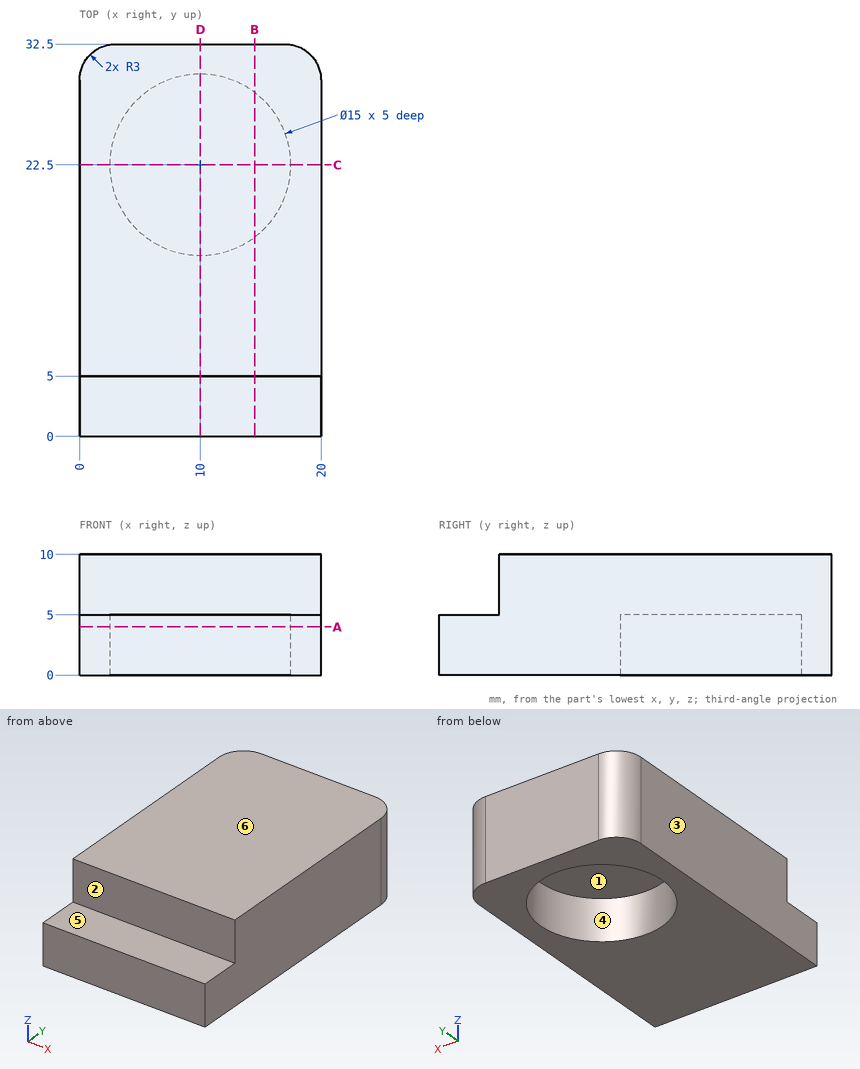
Can you work these out from the drawing? Everything is in mm from the part's minimum corner. A direction names the side the tool comes from. Round coordinates to 2 decimals unless told otherwise and drop trailing zeros. Loops run counter-clockwise (first coordinate to the right, second up) from the corner with the lowest first, then second, coordinate; pieces in that order, holes last. Notation, with made-up numbers: (62.5, 15) -> (96.5, 15) arc R18 cw to (96.5, 43) -> close; hole circle Ø4 at (30.5, -31.75). An arc over 180 degrees is marked (long way). Use CSV: the item, a comma, the result in double quotes.
(1) If we mould it in two halves opening along Y, with no side actions, what happens to the marked faces 1, 2 and 3? For each: +Y half, -Y half, draft (parallel to the pull), parting line (faces both ways), or undercut.
Return value:
face 1,"undercut"
face 2,"-Y half"
face 3,"draft"
(2) Suppose I cut it at C-C on y = 22.5. Write out the boundary of the cut face in (x, z), plus the area to 3 significant figures.
Return value:
outline,"(0, 0) -> (2.5, 0) -> (2.5, 5) -> (17.5, 5) -> (17.5, 0) -> (20, 0) -> (20, 10) -> (0, 10) -> close"
area,"125 mm²"
(3) Suppose I cut it at A-A on z = 4. Write out the boundary of the cut face in (x, y), plus the area to 3 significant figures.
Return value:
outline,"(0, 0) -> (20, 0) -> (20, 29.5) arc R3 ccw to (17, 32.5) -> (3, 32.5) arc R3 ccw to (0, 29.5) -> close; hole circle Ø15 at (10, 22.5)"
area,"469 mm²"
(4) For the marked faces 4, 5 and 6, which set-ups out of +Z, -Z, +X, -X, +Y, -Y let a thin tool reach every point of the face, with its end or its side?
Return value:
face 4,"-Z"
face 5,"+Z, +X, -X, -Y"
face 6,"+Z, +X, -X, +Y, -Y"
(5) If I drill on probe 1 along Y at (x, z) = (10, 2.35); probe 2 along Z at (x, y) = (14.25, 24.5); probe 3 along X at (y, z) = (23, 3), over which ranges is the centre line in solid material (lowest first)? Write a range as [from, to].
Return value:
probe 1,"y = [0, 15], [30, 32.5]"
probe 2,"z = [5, 10]"
probe 3,"x = [0, 2.52], [17.48, 20]"
(6) Suppose I cut it at D-D on x = 10. Write out the boundary of the cut face in (y, z), plus the area to 3 significant figures.
Return value:
outline,"(0, 0) -> (15, 0) -> (15, 5) -> (30, 5) -> (30, 0) -> (32.5, 0) -> (32.5, 10) -> (5, 10) -> (5, 5) -> (0, 5) -> close"
area,"225 mm²"
(7) Will these pins go through, and if not, where does the flat tip stop? pin 1 Ø12 at (x, y) = (10, 22.5) entering from -Z; pin 2 Ø4 at (x, z) = (11.5, 7.5) entering from -Y.
Return value:
pin 1,"stops at z = 5"
pin 2,"stops at y = 5"
(8) Suppose I cut it at B-B on x = 14.5. Write out the boundary of the cut face in (y, z).
Return value:
outline,"(0, 0) -> (16.5, 0) -> (16.5, 5) -> (28.5, 5) -> (28.5, 0) -> (32.5, 0) -> (32.5, 10) -> (5, 10) -> (5, 5) -> (0, 5) -> close"
